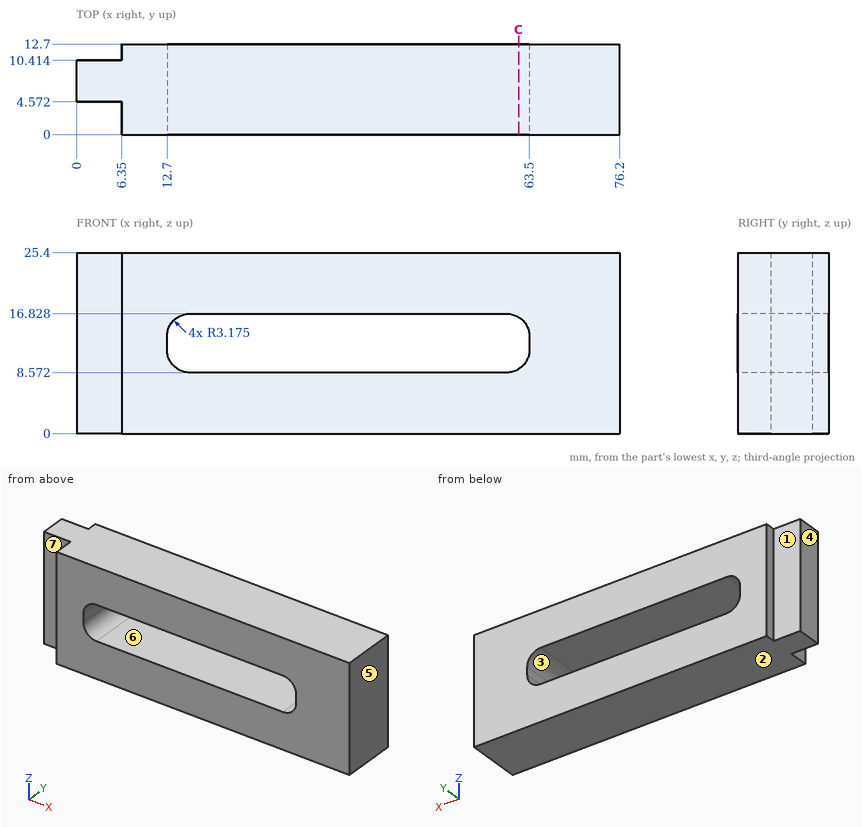
Job drawing, mm, ordinate dimensions from the low corner. One solid piece. A direction names the side the tool comes from. Give positions to 0.01 mm unless a question says otherwise; leave off trailing zeros. Write each loop counter-clockwise with the first axis right and the second up, starting at its lowest first coordinate (ties: lowest second). Pieces come first, ordered by that corner, then holes. Notation, with made-up numbers: (71.5, 7) - (84.5, 7) arc R33 ccw to (84.5, 44) - close; hole circle Ø9 at (23.25, 79.5). An arc over 180 degrees is marked (long way). Use one line per item in the form item = value. Start each with the question number.
1. Band-saw the part on C-C on x = 62. Write the cut outline in (y, z).
2. Probe line 1 (Z direction, x = 17.5, y = 10); line 2 (X direction, y = 10.25, z = 13); line 3 (X direction, y = 2.5, z = 4.5). List the from-to ranges inside material, lowest first. Write a range as [from, to].
3. 3-axis set-ups, long thin cutter, end or side, ignore diameter. For the marked faces 1, 2 and 3: which of +Z, -Z, +X, -X, +Y, -Y reach the whole face in a straight line?
4. Drop flat-ended pins along their axis: pin 1 Ø1.9 at (x, z) = (3.5, 12.5) entering from -Y; pin 2 Ø1.4 at (y, z) = (2, 16) entering from -X; pin 3 Ø1.8 at (y, z) = (12, 9) entering from -X. Give the stop position or say it passes through.
5. Two-plate mould, pull along X, no slides. Class the marked faces 4, 5, 6 and 7: released by +X, released by -X, zero draft, split by the parting line, or undercut.
Conclusion:
q1.outline = (0, 0) - (12.7, 0) - (12.7, 9.05) - (0, 9.05) - close; (0, 16.35) - (12.7, 16.35) - (12.7, 25.4) - (0, 25.4) - close
q2.line_1 = [0, 8.57], [16.83, 25.4]
q2.line_2 = [0, 12.7], [63.5, 76.2]
q2.line_3 = [6.35, 76.2]
q3.face_1 = +Z, -Z, -X, +Y
q3.face_2 = -Z, +X, -X, +Y, -Y
q3.face_3 = +Y, -Y
q4.pin_1 = 4.57
q4.pin_2 = 6.35
q4.pin_3 = 6.35
q5.face_4 = released by -X
q5.face_5 = released by +X
q5.face_6 = undercut
q5.face_7 = zero draft
